```python
from build123d import *

# Parameters (mm, degrees)
F1_DEPTH = 11
F3_DEPTH = 11
F5_DEPTH = 4


with BuildPart() as f1:
    # F0 (on Front) → F1 (new body)
    with BuildSketch(Plane.XZ):
        with BuildLine():
            Line((-19, 38), (-19, 0))
            Line((-19, 0), (19, 0))
            Line((19, 0), (19, 38))
            ThreePointArc((19, 38), (0, 57), (-19, 38))
        make_face()
    extrude(amount=F1_DEPTH)

    # F2 (on Top) → F3 (join)
    with BuildSketch(Plane.XY):
        with BuildLine():
            Line((19, 0), (-19, 0))
            Line((-19, 0), (-19, -38))
            ThreePointArc((-19, -38), (0, -57), (19, -38))
            Line((19, -38), (19, 0))
        make_face()
    extrude(amount=F3_DEPTH)

    # F4 (on Right) → F5 (join)
    with BuildSketch(Plane.YZ):
        Polygon((-11, 49), (-49, 11), (-11, 9.028562), align=None)
    extrude(amount=F5_DEPTH)

    # F6: F1 across plane


with BuildPart() as f1_1:
    add(f1.part)
    add(f1.part.mirror(Plane.YZ))


solid = f1_1.part
```
Build history of the part. All positions in model axes, mm. A direction names the side the tool comes from. Coordinates: 2 decimals unless noted, no trailing zeros. Write each loop counter-clockwise with the first axis right and the second up, starting at its lowest first coordinate (ties: lowest second). Pieces come first, ordered by that corner, then holes.
1. Band-saw the part on C-C, the plane x = 0. Give the cut face in (y, z), and give its area (4 significant figures).
Answer block:
outline: (-57, 0) - (0, 0) - (0, 57) - (-11, 57) - (-11, 49) - (-49, 11) - (-57, 11) - close
area: 1,855 mm2
2. Band-saw the part on D-D, the plane x = -17. Give the cut face in (y, z), and give its area (3 significant figures).
Answer block:
outline: (-46.49, 0) - (0, 0) - (0, 46.49) - (-11, 46.49) - (-11, 11) - (-46.49, 11) - close
area: 902 mm2
3. 3-axis set-ups, long thin cutter, end or side, ignore diameter. For faces 1 (the flat face through (0, 0, 29)), 2 (the flat face through (4, -22, 22)), 3 (the flat face through (-4.5, -33.7, 11)), 4 (the flat face through (-4, -22, 22)), 5 (the flat face through (-19, -10, 15)): which of +Z, -Z, +X, -X, +Y, -Y reach the whole face in a straight line?
Answer block:
face 1: +Z, -Z, +X, -X, +Y
face 2: +Z, +X, -Y
face 3: +Z, -Y
face 4: +Z, -X, -Y
face 5: +Z, -Z, -X, +Y, -Y
4. Band-saw the part on B-B, the plane y = -20. Give the cut face in (x, z), and give its area (3 significant figures).
Answer block:
outline: (-19, 0) - (19, 0) - (19, 11) - (4, 11) - (4, 40) - (-4, 40) - (-4, 11) - (-19, 11) - close
area: 650 mm2
5. Drop flat-ended pins along their axis: pin 1 (1.5 mm diameter, centred on x = -5.5, z = 8, fed in from -Y); pin 2 (11.5 mm diameter, centred on y = -26, z = 25.5, fed in from -X); pin 3 (19 mm diameter, centred on y = -21, z = 26.5, fed in from +X). Give the stop position or say it passes through.
Answer block:
pin 1: stops at y = -56.4
pin 2: stops at x = -4
pin 3: stops at x = 4
6. Drill centre lines: probe 1 along Y at (x, z) = (16, 40.5); probe 2 along Z at (x, y) = (13, -46); probe 3 along X at (y, z) = (-21.5, 15.5). Where is each one in solid material? Low to high.
Answer block:
probe 1: y = -11 to 0
probe 2: z = 0 to 11
probe 3: x = -4 to 4
7. Band-saw the part on A-A, the plane z = 17.5. Give the cut face in (x, y), and give its area (3 significant figures).
Answer block:
outline: (-19, -11) - (-4, -11) - (-4, -42.5) - (4, -42.5) - (4, -11) - (19, -11) - (19, 0) - (-19, 0) - close
area: 670 mm2
